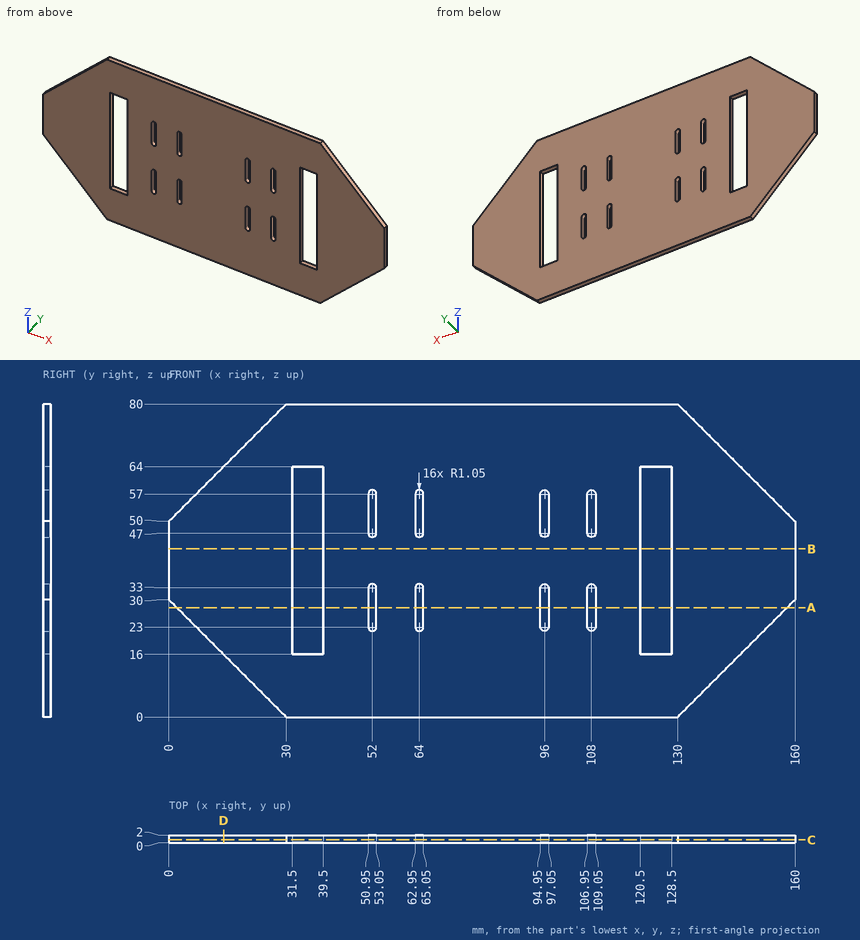
Print and shaded views of the part. All mm, measured from the part's lowest x, y and z. Give positions to 0.01 mm unless a question says otherwise; leave off trailing zeros. Loops run counter-clockwise (first coordinate to the right, second up) from the corner with the lowest first, then second, coordinate; pieces in that order, holes last. Notation, with made-up numbers: (10.25, -10) -> (23.25, -10) arc R32 ccw to (23.25, 16) -> close; hole circle Ø9 at (60, -13.5). An arc over 180 degrees is marked (long way). One line per question, with ' | ' between items. Start each with the question number.
1) Probe L1, parallel to X at y = 0.6, z = 44.5; L2, parallel to X at y = 1.95, z = 21.5; L3, parallel to Z at x = 153, y = 1.2. List the from-to ranges inside material, lowest first.
2) Cut at D-D (x = 14). Give the cut face in (y, z).
3) Cut at B-B (z = 43). Give the cut face in (x, y), plus the area to 3 significant figures.
4) Cut at A-A (z = 28). Give the cut face in (x, y).
5) Cut at C-C (y = 0.8). Count the separate pieces of the cut face and the enclosed holes in it, plus the area to 3 significant figures.
6) Pin check, flat tips, straight feed: pin 1 (1 mm diameter, centred on y = 1, z = 28.5, fed in from +X); pin 2 (1 mm diameter, centred on y = 1, z = 25.5, fed in from -X); pin 3 (0.6 mm diameter, centred on y = 0.5, z = 26, fed in from +X). Stop position of each tip, or through.
Return value:
1) L1: 0 to 31.5, 39.5 to 120.5, 128.5 to 160 | L2: 8.5 to 31.5, 39.5 to 120.5, 128.5 to 151.5 | L3: 23 to 57
2) outline: (0, 16) -> (2, 16) -> (2, 64) -> (0, 64) -> close
3) outline: (0, 0) -> (31.5, 0) -> (31.5, 2) -> (0, 2) -> close; (39.5, 0) -> (120.5, 0) -> (120.5, 2) -> (39.5, 2) -> close; (128.5, 0) -> (160, 0) -> (160, 2) -> (128.5, 2) -> close | area: 288 mm^2
4) outline: (2, 0) -> (31.5, 0) -> (31.5, 2) -> (2, 2) -> close; (39.5, 0) -> (50.95, 0) -> (50.95, 2) -> (39.5, 2) -> close; (53.05, 0) -> (62.95, 0) -> (62.95, 2) -> (53.05, 2) -> close; (65.05, 0) -> (94.95, 0) -> (94.95, 2) -> (65.05, 2) -> close; (97.05, 0) -> (106.95, 0) -> (106.95, 2) -> (97.05, 2) -> close; (109.05, 0) -> (120.5, 0) -> (120.5, 2) -> (109.05, 2) -> close; (128.5, 0) -> (158, 0) -> (158, 2) -> (128.5, 2) -> close
5) separate pieces: 1 | enclosed holes: 10 | area: 10,000 mm^2
6) pin 1: x = 159 | pin 2: x = 4 | pin 3: x = 156.3
